Geometry: final body of the model. Coordinates: model frame, mm. A direction names the side the tool comes from. Round coordinates to 2 decimals unless told otherwise and drop trailing zeros. Write each loop counter-clockwise with the first axis right and the second up, starting at its lowest first coordinate (ties: lowest second). Pieces come first, ordered by that corner, then holes. Notation, with made-up numbers: M 74,53.5 L 89,53.5 A14 ccw 89,64.5 Z; hole C 23.5,38.25 d8. An arc over 180 degrees is marked long. Use one line per item in the form item = value. Start each with the question number.
Item 1: Pull-direction query (X, two-part tool) for faces 4 (the flat face through (24.697, 39, 5)), 5 (the flat face through (32, 43.586, 5)), 6 (the flat face through (40.697, 39, 5)); classes: pulls with the +X half, pulls with the -X half, needs draft (parallel to the pull), parting line crosses it, or undercut.
Item 2: Ray query, probe 1 along Y at (x, z) = (31.5, 8.5); probe 2 along X at (y, z) = (39, 7.25); probe 3 along X at (y, z) = (42, 5.5). Return the intervals inside material, ascending.
Item 3: Section query B-B (z = 2.5). Return loops of the section in (x, y).
Item 4: Section query A-A (x = 28.75). Return loops of the section in (y, z), and give its area (3 significant figures).
Item 5: Section query C-C (y = 39.25). Return loops of the section in (x, z).
Item 6: Section query D-D (x = 33). Return loops of the section in (y, z).
Item 7: Reachability of faces 1 (the cylindrical face through (36.156, 42.107, 4.722)), 2 (the flat face through (34.1, 40.586, 2.7)), 3 (the flat face through (43.697, 39, 5)) from +Z, -Z, +X, -X, +Y, -Y: full face, straight path, thin tool, end or side. Return the list, or none.
from build123d import *

# Parameters (mm, degrees)
SKETCH3_W           = 19
SKETCH3_H           = 10
SKETCH3_W_2         = 13
SKETCH3_H_2         = 4
BOSS_EXTRUDE1_DEPTH = 10
SKETCH4_R           = 2
CUT_EXTRUDE1_DEPTH  = 4


with BuildPart() as part:
    # Sketch3 → Boss-Extrude1 (new body)
    with BuildSketch(Plane.XY):
        with Locations((34.196690887, 38.585532183)):
            Rectangle(SKETCH3_W, SKETCH3_H)
        with Locations((34.196690887, 38.585532183)):
            Rectangle(SKETCH3_W_2, SKETCH3_H_2, mode=Mode.SUBTRACT)
    extrude(amount=BOSS_EXTRUDE1_DEPTH)

    # Sketch4 → Cut-Extrude1 (cut)
    with BuildSketch(Plane(origin=(0, 43.585532183, 0), x_dir=(1, 0, 0), z_dir=(0, 1, 0))):
        with Locations(Location((34.172706418, -4.982011648, 0), (0, 0, 270))):
            Circle(SKETCH4_R)
    extrude(amount=-CUT_EXTRUDE1_DEPTH, mode=Mode.SUBTRACT)


solid = part.part
Working result:
q1.face_4 = pulls with the -X half
q1.face_5 = needs draft
q1.face_6 = undercut
q2.probe_1 = 33.59 to 36.59, 40.59 to 43.59
q2.probe_2 = 24.7 to 27.7, 40.7 to 43.7
q2.probe_3 = 24.7 to 32.24, 36.1 to 43.7
q3.outline = M 24.7,33.59 L 43.7,33.59 L 43.7,43.59 L 24.7,43.59 Z; hole M 27.7,36.59 L 40.7,36.59 L 40.7,40.59 L 27.7,40.59 Z
q4.outline = M 33.59,0 L 36.59,0 L 36.59,10 L 33.59,10 Z; M 40.59,0 L 43.59,0 L 43.59,10 L 40.59,10 Z
q4.area = 60.0 mm²
q5.outline = M 24.7,0 L 27.7,0 L 27.7,10 L 24.7,10 Z; M 40.7,0 L 43.7,0 L 43.7,10 L 40.7,10 Z
q6.outline = M 33.59,0 L 36.59,0 L 36.59,10 L 33.59,10 Z; M 40.59,0 L 43.59,0 L 43.59,3.36 L 40.59,3.36 Z; M 40.59,6.6 L 43.59,6.6 L 43.59,10 L 40.59,10 Z
q7.face_1 = +Y
q7.face_2 = +Z, -Z
q7.face_3 = +Z, -Z, +X, +Y, -Y
